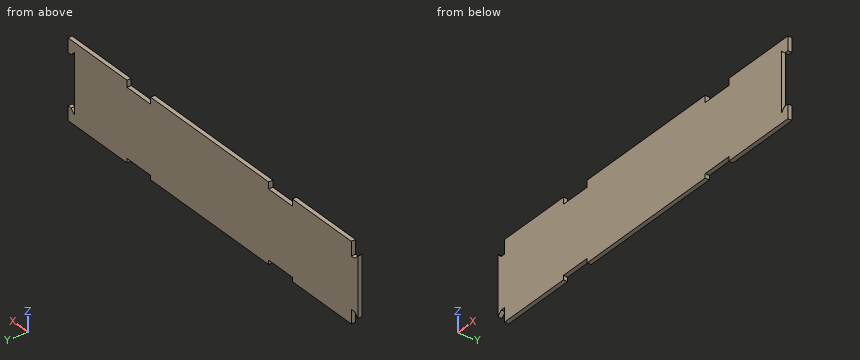
```python
from build123d import *

# Parameters (mm, degrees)
F0_W     = 278.2466876
F0_H     = 50.8
F1_DEPTH = 3.175
F2_W     = 57.9247
F2_H     = 5.08
F2_W_2   = 115.8494
F2_H_2   = 3.1496
F3_DEPTH = 3.175
F5_DEPTH = 3.175
F6_DEPTH = 3.176


with BuildPart() as f1:
    # F0 (on Front) → F1 (new body)
    with BuildSketch(Plane.XZ):
        with Locations((139.1233438, 25.4)):
            Rectangle(F0_W, F0_H)
    extrude(amount=F1_DEPTH)

    # F2 (on face) → F3 (join)
    with BuildSketch(Plane.XZ.offset(3.175)):
        with Locations((28.96235, 53.34)):
            Rectangle(F2_W, F2_H)
        with Locations((139.1233438, 53.34)):
            Rectangle(F2_W_2, F2_H)
        with Locations((249.2843376, 53.34)):
            Rectangle(F2_W, F2_H)
        with Locations((28.96235, -1.5748)):
            Rectangle(F2_W, F2_H_2)
        with Locations((139.1233438, -1.5748)):
            Rectangle(F2_W_2, F2_H_2)
        with Locations((249.2843376, -1.5748)):
            Rectangle(F2_W, F2_H_2)
    extrude(amount=-F3_DEPTH)

    # F4 (on face) → F5 (join)
    with BuildSketch(Plane.XZ.offset(3.175)):
        Polygon((0, 7.3152), (0, 45.4152), (-3.175, 45.4152), (-6.35, 48.5902), (-6.35, 4.1402), (-3.175, 7.3152), align=None)
    extrude(amount=-F5_DEPTH)

    # F4 (on face) → F6 (cut, through all)
    with BuildSketch(Plane.XZ.offset(3.175)):
        Polygon((278.2466876, 7.3152), (278.2466876, 45.4152), (275.0716876, 45.4152), (271.8966876, 48.5902), (271.8966876, 4.1402), (275.0716876, 7.3152), align=None)
    extrude(amount=-F6_DEPTH, mode=Mode.SUBTRACT)


solid = f1.part
```
The model under review builds one solid part; all positions refer to its coordinate system, in mm. Round coordinates to 2 decimals unless told otherwise and drop trailing zeros. Write each loop counter-clockwise with the first axis right and the second up, starting at its lowest first coordinate (ties: lowest second). Pieces come first, ordered by that corner, then holes. Notation, with made-up numbers: (-37.5, -26.75) -> (-8.5, -26.75) arc R26 ccw to (-8.5, -11.75) -> close; hole circle Ø8 at (18.25, 36). An arc over 180 degrees is marked (long way). Use CSV: the item, a comma, the result in double quotes.
Q1. To check wall thickness, follow probe 1 along X at (y, z) = (-1.1, 51.5); probe 2 along X at (y, z) = (-1.1, 46); probe 3 along X at (y, z) = (-0.2, 1.5). State the ranges of each line that lie inside material, in increasing order. Write a range as [from, to].
Checks:
probe 1,"[0, 57.92], [81.2, 197.05], [220.32, 278.25]"
probe 2,"[-6.35, -3.76], [0, 271.9], [274.49, 278.25]"
probe 3,"[0, 278.25]"
Q2. For pin 1 Ø1.6 at (x, y) = (66.5, -1) entering from -Z; pin 2 Ø1.6 at (y, z) = (-2.5, 53) entering from -X; pin 3 Ø1.6 at (x, y) = (-1, -1.5) entering from -Z, all flat-tipped, find the tip position at first contact; note any pin that passes through.
Checks:
pin 1,"z = 0"
pin 2,"x = 0"
pin 3,"z = 7.32"
Q3. Consider section B-B (x = 215). Give the boundary of the cut face in (y, z) (3 decimals), then the cut area to 3 significant figures.
Checks:
outline,"(-3.175, 0) -> (0, 0) -> (0, 50.8) -> (-3.175, 50.8) -> close"
area,"161 mm²"
Q4. Consider section C-C (z = 28.5). Give the boundary of the cut face in (x, y) (3 decimals), then the cut area to 3 significant figures.
Checks:
outline,"(-6.35, -3.175) -> (271.897, -3.175) -> (271.897, 0) -> (-6.35, 0) -> close"
area,"883 mm²"
